```python
from build123d import *

# Parameters (mm, degrees)
SKETCH1_W           = 168.65
SKETCH1_H           = 208.65
BOSS_EXTRUDE1_DEPTH = 3.18
CUT_EXTRUDE1_REACH  = 136.181
CUT_EXTRUDE24_REACH = 136.181
SKETCH45_R          = 25.951103398


with BuildPart() as part:
    # Sketch1 → Boss-Extrude1 (new body)
    with BuildSketch(Plane(origin=(0, 0, 0), x_dir=(1, 0, 0), z_dir=(0, 1, 0))):
        Rectangle(SKETCH1_W, SKETCH1_H)
    extrude(amount=BOSS_EXTRUDE1_DEPTH)

    # Sketch2 → Cut-Extrude1 (cut, up to next)
    with BuildSketch(Plane(origin=(0, 3.18, 0), x_dir=(1, 0, 0), z_dir=(0, 1, 0)), mode=Mode.PRIVATE) as cut_extrude1_sk1:
        with BuildLine():
            Line((10.675, -56.675), (-9.325, -56.675))
            ThreePointArc((-9.325, -56.675), (-11.825, -59.175), (-9.325, -61.675))
            Line((-9.325, -61.675), (10.675, -61.675))
            ThreePointArc((10.675, -61.675), (13.175, -59.175), (10.675, -56.675))
        make_face()
    cut_extrude1_tool1 = extrude(cut_extrude1_sk1.sketch, amount=-CUT_EXTRUDE1_REACH, mode=Mode.PRIVATE) & part.part
    add(cut_extrude1_tool1.solids().sort_by_distance((0.675, 3.18, 59.175))[0], mode=Mode.SUBTRACT)

    # Sketch45 → Cut-Extrude24 (cut, up to next)
    with BuildSketch(Plane(origin=(0, 3.18, 0), x_dir=(1, 0, 0), z_dir=(0, 1, 0)), mode=Mode.PRIVATE) as cut_extrude24_sk1:
        with Locations(Location((-42.4825, 0, 0), (0, 0, 270))):
            Circle(SKETCH45_R)
    cut_extrude24_tool1 = extrude(cut_extrude24_sk1.sketch, amount=-CUT_EXTRUDE24_REACH, mode=Mode.PRIVATE) & part.part
    add(cut_extrude24_tool1.solids().sort_by_distance((-42.4825, 3.18, 0))[0], mode=Mode.SUBTRACT)


solid = part.part
```
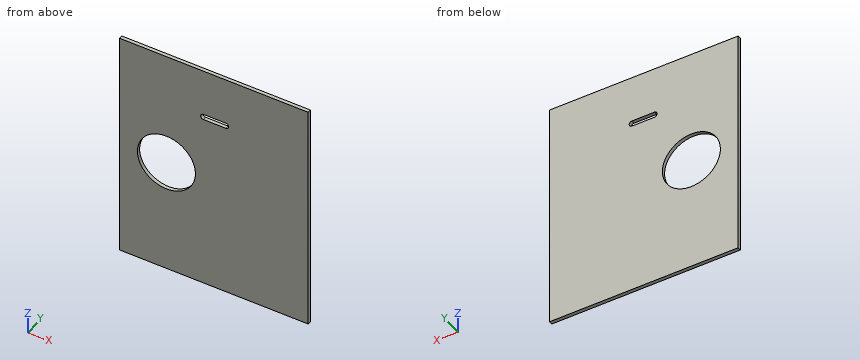
Geometry check sheet. Reference: the model listing, model coordinates, mm. Coordinates: 2 decimals unless noted, no trailing zeros. Order: outer loops, then holes, each group sorted by start corner. A loop starts at its lowest first (then second) coordinate and runs counter-clockwise, first axis right, second up.
Item 1: Section check C-C (y = 2.15). Enter the section's corners in (x, z) (1 decimal), plus the area to 3 significant figures.
Item 2: Scan lines: line 1 along X through (y, z) = (0.75, 0) (3 decimals); line 2 along Z through (x, y) = (-4, 2.25) (3 decimals); line 3 along Z through (x, y) = (-41.5, 1.05) (1 decimal). Record each from-to range of solid material in increasing order.
Item 3: Section check A-A (z = 0). Enter the section's corners in (x, y) (3 decimals).
Item 4: Section check B-B (x = -60.5). Enter the section's corners in (y, z) (3 decimals).
Check sheet entries:
1. outline: (-84.3, -104.3) - (84.3, -104.3) - (84.3, 104.3) - (-84.3, 104.3) - close; hole circle Ø51.9 at (-42.5, 0); hole (-9.3, 56.7) - (10.7, 56.7) arc R2.5 ccw to (10.7, 61.7) - (-9.3, 61.7) arc R2.5 ccw to start
1. area: 33,000 mm2
2. line 1: x = -84.325 to -68.434, -16.531 to 84.325
2. line 2: z = -104.325 to 56.675, 61.675 to 104.325
2. line 3: z = -104.3 to -25.9, 25.9 to 104.3
3. outline: (-84.325, 0) - (-68.434, 0) - (-68.434, 3.18) - (-84.325, 3.18) - close; (-16.531, 0) - (84.325, 0) - (84.325, 3.18) - (-16.531, 3.18) - close
4. outline: (0, -104.325) - (3.18, -104.325) - (3.18, -18.677) - (0, -18.677) - close; (0, 18.677) - (3.18, 18.677) - (3.18, 104.325) - (0, 104.325) - close
